Here's the drawing with two shaded views (mm, measured from the low corner). I have some questions. Give positions to 0.01 mm unless a question says otherwise; leave off trailing zeros. Loops run counter-clockwise (first coordinate to the right, second up) from the corner with the lowest first, then second, coordinate; pieces in that order, holes last. Notation, with made-up numbers: M 0.5,34 L 26.5,34 A12 ccw 26.5,44 Z; hole C 26.25,58 d5. An arc over 180 degrees is marked long. Use CSV: the item, a comma, the result in double quotes.
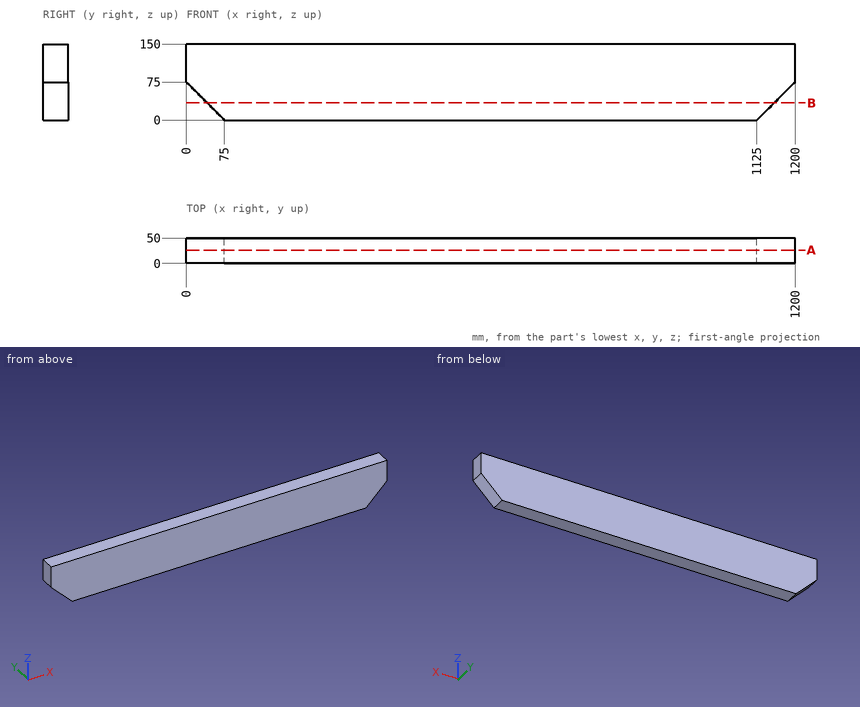
1. I want a section at A-A, the plane y = 26. List the corners of the cut face in (x, z) for me, then the cut area to 3 significant figures.
Outcome:
outline,"M 0,75 L 75,0 L 1125,0 L 1200,75 L 1200,150 L 0,150 Z"
area,"174,000 mm2"
2. Please list where these lines run through material, in increasing order: line 1 (X direction, y = 16, z = 49.5); line 2 (X direction, y = 40, z = 58).
Outcome:
line 1,"25.5 to 1174.5"
line 2,"17 to 1183"
3. I want a section at B-B, the plane z = 34. List the corners of the cut face in (x, y) for me.
Outcome:
outline,"M 41,0 L 1159,0 L 1159,50 L 41,50 Z"
